Autodesk Inventor part; units mm, degrees
ref_plane "Flange Pattern Plane" through (19.05, 7.9375, -4.5466) normal (0, 1, 0) x (1, 0, 0)
ref_plane "YZ Plane" through (0, 0, 0) normal (1, 0, 0) x (0, 1, 0)
ref_plane "XZ Plane" through (0, 0, 0) normal (0, 1, 0) x (-1, 0, 0)
sketch "Sketch1" plane through (0, 0, 0) normal (0, 1, 0) x (-1, 0, 0)
  line L0 (-19.05, 0) -> (19.05, 0)
  line L1 (19.05, 0) -> (19.05, -25.4)
  line L2 (19.05, -25.4) -> (-19.05, -25.4)
  line L3 (-19.05, -25.4) -> (-19.05, 0)
  line L4 (19.05, 0) -> (-19.05, -25.4) construction
  point P0 (0, 0)
  point P1 (0, 0)
  dimension "d0" = 38.1
  dimension "d1" = 25.4
extrude "Plate1" add sketch "Sketch1" along normal blind 1.5875
sketch "Sketch2" plane through (17.4625, 0, -25.4) normal (1, 0, 0) x (0, 1, 0)
  line L0 (0, 25.4) -> (0, 0)
  line L1 (0, 0) -> (14.2875, 0)
  line L2 (14.2875, 0) -> (14.2875, 25.4)
  line L3 (14.2875, 25.4) -> (0, 25.4)
edge flange "Flanges" height 12.7 angle 90 thickness 1.5875 bend radius 0.7937 thickness toward (1, 0, 0) relief tear relief width 1.5875 relief depth 0.7937 corner gap 1.5875 corner form 0 edges at (19.05, 1.5875, -12.7) (-19.05, 1.5875, -12.7) wall of the first edge with corners at (17.4625, 0, 0) (17.4625, 0, -25.4) (17.4625, 14.2875, -25.4) (17.4625, 14.2875, 0)
bend "Bend1"
corner "Corner1"
sketch "Sketch3" plane through (19.05, 2.3813, -25.4) normal (1, 0, 0) x (0, 0, -1)
  line L0 (-20.8534, 7.8677) -> (-17.2466, 7.8677)
  line L1 (-16.7386, 7.3597) -> (-16.7386, 3.7529)
  line L2 (-17.2466, 3.2449) -> (-20.8534, 3.2449)
  line L3 (-21.3614, 3.7529) -> (-21.3614, 7.3597)
  arc A0 (-20.8534, 7.8677) -> (-21.3614, 7.3597) centre (-20.8534, 7.3597) ccw
  arc A1 (-16.7386, 7.3597) -> (-17.2466, 7.8677) centre (-17.2466, 7.3597) ccw
  arc A2 (-17.2466, 3.2449) -> (-16.7386, 3.7529) centre (-17.2466, 3.7529) ccw
  arc A3 (-21.3614, 3.7529) -> (-20.8534, 3.2449) centre (-20.8534, 3.7529) ccw
  line L4 (-25.4, 0) -> (-25.4, 11.9063) construction
  line L5 (-25.4, 11.9063) -> (0, 11.9062) construction
  line L6 (-20.8534, 7.3597) -> (-17.2466, 3.7529) construction
  point P0 (-25.4, -2.3812)
  point P1 (-16.7386, 3.2449)
  point P2 (-21.3614, 3.2449)
  point P3 (-19.05, 5.5563)
  dimension "d16" = 4.6228
  dimension "d17" = 0.508
  dimension "d20" = 6.35
  dimension "d21" = 6.35
extrude "Flange Stamp" cut sketch "Sketch3" against normal blind 1.5875
sketch "Sketch7" plane through (19.05, 2.3813, 0) normal (1, 0, 0) x (0, 0, -1)
  arc A0 (4.5466, 7.8677) -> (4.0386, 7.3597) centre (4.5466, 7.3597) ccw construction
  arc A1 (8.1534, 3.2449) -> (8.6614, 3.7529) centre (8.1534, 3.7529) ccw construction
  circle A2 centre (6.35, 5.5563) radius 2.1844
  line L0 (4.5466, 7.3597) -> (8.1534, 3.7529) construction
  point P0 (0, -2.3812)
  dimension "d46" = 4.3688
surface extrude "Flange Circle" sketch "Sketch7" against normal up to surface (1.5875 mm away) shown yes curves A2
ref_plane "Flange Pattern Plane" through (19.05, 7.9375, -4.5466) normal (0, 1, 0) x (1, 0, 0)
sketch "Flange Pattern Sketch" plane through (19.05, 7.9375, -4.5466) normal (0, 1, 0) x (1, 0, 0)
  line L0 (0, 3.6068) -> (0, 0) construction
  line L1 (-45.8186, -4.5466) -> (8.2118, -4.5466) construction
  line L2 (0, 0) -> (-1.5875, 0) construction
  point P0 (-19.05, -4.5466)
  point P1 (0, 1.8034)
  point P2 (0, 14.5034)
  dimension "d131" = 12.7
  dimension "d134" = 12.7
pattern_sketch "Flange Pattern" of "Flange Circle", "Flange Stamp" from (19.05, 7.9375, -6.35) copies at (19.05, 7.9375, -19.05)
sketch "Sketch8" plane through (0, 0, 0) normal (0, -1, 0) x (1, 0, 0)
  line L0 (16.6687, 0) -> (-16.6687, 0) construction
  line L1 (14.5034, -4.0386) -> (10.8966, -4.0386)
  line L2 (10.3886, -4.5466) -> (10.3886, -8.1534)
  line L3 (10.8966, -8.6614) -> (14.5034, -8.6614)
  line L4 (15.0114, -8.1534) -> (15.0114, -4.5466)
  arc A0 (15.0114, -4.5466) -> (14.5034, -4.0386) centre (14.5034, -4.5466) ccw
  arc A1 (14.5034, -8.6614) -> (15.0114, -8.1534) centre (14.5034, -8.1534) ccw
  arc A2 (10.3886, -8.1534) -> (10.8966, -8.6614) centre (10.8966, -8.1534) ccw
  arc A3 (10.8966, -4.0386) -> (10.3886, -4.5466) centre (10.8966, -4.5466) ccw
  line L5 (14.5034, -4.5466) -> (10.8966, -8.1534) construction
  line L6 (19.05, 0) -> (19.05, -25.4) construction
  point P0 (0, 0)
  point P1 (10.3886, -8.6614)
  point P2 (15.0114, -8.6614)
  point P3 (12.7, -6.35)
  dimension "d49" = 4.6228
  dimension "d50" = 0.508
  dimension "d51" = 6.35
  dimension "d52" = 6.35
extrude "Body Stamp" cut sketch "Sketch8" against normal blind 1.5875
sketch "Sketch9" plane through (0, 0, 0) normal (0, -1, 0) x (1, 0, 0)
  arc A0 (15.0114, -4.5466) -> (14.5034, -4.0386) centre (14.5034, -4.5466) ccw construction
  arc A1 (10.3886, -8.1534) -> (10.8966, -8.6614) centre (10.8966, -8.1534) ccw construction
  line L0 (14.5034, -4.5466) -> (10.8966, -8.1534) construction
  circle A2 centre (12.7, -6.35) radius 2.1844
  point P0 (0, 0)
  dimension "d55" = 4.3688
surface extrude "Body Circle" sketch "Sketch9" against normal up to surface (1.5875 mm away) shown yes curves A2
sketch "Body Pattern Sketch" plane through (0, 0, 0) normal (0, -1, 0) x (1, 0, 0)
  line L0 (16.6687, 0) -> (-16.6687, 0) construction
  line L1 (19.05, 0) -> (19.05, -25.4) construction
  circle A0 centre (12.7, -6.35) radius 2.1844 construction
  point P0 (0, 0)
  point P1 (12.7, -19.05)
  dimension "d62" = 12.7
  dimension "d65" = 12.7
  dimension "d139" = 12.7
pattern_sketch "Body Pattern" of "Body Stamp", "Body Circle" from (12.7, 0, -6.35) copies at (12.7, 0, -19.05)
sketch "Arc Length" plane through (17.4625, 2.3813, 0) normal (0, 0, 1) x (1, 0, 0)
  line L0 (0, 0) -> (1.5875, 0) construction
  arc A0 (-0.7937, -0.7938) -> (0, 0) centre (-0.7937, 0) ccw construction
  line L1 (-0.7938, -2.3813) -> (-0.7937, -0.7938) construction
  arc A1 (-0.7938, -2.3813) -> (1.5875, 0) centre (-0.7937, 0) ccw construction
  point P0 (-17.4625, -2.3812)
  dimension "d85" = 3.7405
  dimension "d92" = 1.2468
sketch "Sketch13" plane through (19.05, 14.2875, 0) normal (1, 0, 0) x (0, 0, -1)
  line L0 (0, 0) -> (25.4, 0) construction
  line L1 (62.4078, 0) -> (63.4238, -1.016)
  line L2 (63.4238, -1.016) -> (64.4398, 0)
  line L3 (62.4078, 0) -> (64.4398, 0)
  line L4 (25.4, -11.9062) -> (0, -11.9062) construction
  line L5 (63.4238, -10.8903) -> (61.161, -13.1531)
  line L6 (61.161, -13.1531) -> (63.4238, -15.4159)
  line L7 (63.4238, -15.4159) -> (65.6866, -13.1531)
  line L8 (65.6866, -13.1531) -> (63.4238, -10.8903)
  line L9 (63.4238, -10.8903) -> (63.4238, -15.4159) construction
  line L10 (63.4238, -1.016) -> (63.4238, -10.8903) construction
  line L11 (0, -11.9062) -> (25.4, -11.9062) construction
  point P0 (0, -14.2875)
  dimension "d86" = 4.5256
  dimension "d88" = 1.016
  dimension "d91" = 1.016
  dimension "d102" = 63.4238
feature "Notch" [suppressed]
mirror "Notch Mirror" [suppressed]
pattern_linear "Notch Pattern" [suppressed]
chamfer "End Chamfer" distance 1.016 angle 45 4 edges at (-18.2562, 14.2875, -25.4) (18.2563, 14.2875, -25.4) (-18.2562, 14.2875, 0) (18.2562, 14.2875, 0)
sketch "Sketch14" plane through (-19.05, 2.3813, 419.1) normal (1, 0, 0) x (0, 0, -1)
  line L0 (419.1, 11.9063) -> (444.5, 11.9063) construction
  line L1 (419.1, 0) -> (419.1, 11.9063) construction
  line L2 (419.1, -2.3813) -> (444.5, -2.3813) construction
  line L3 (419.1, 11.9063) -> (444.5, 11.9063)
  line L4 (444.5, 11.9063) -> (444.5, -2.3813)
  line L5 (444.5, -2.3813) -> (419.1, -2.3813)
  line L6 (419.1, -2.3813) -> (419.1, 11.9063)
  point P0 (419.1, -2.3812)
  point P1 (382.0521, -1.9844)
extrude "Half Cut" cut sketch "Sketch14" along normal blind 25.4
equation "\"d1\" = 1.27 * Length"
equation "\"d18\" = Thickness"
equation "\"d53\" = Thickness"
equation "\"d89\" = Thickness"
equation "\"d2\" = Thickness"
equation "\"d3\" = BendReliefWidth"
equation "\"d4\" = BendReliefDepth"
equation "\"d5\" = MinimumRemnant"
equation "\"d6\" = TransitionRadius"
equation "\"d10\" = CornerReliefSize"
equation "\"d11\" = GapSize"
equation "\"d12\" = JacobiRadiusSize"
equation "\"BendRadius\" = Thickness"
equation "\"BendReliefWidth\" = Thickness"
equation "\"BendReliefDepth\" = 0.5 * Thickness"
equation "\"CornerReliefSize\" = 4 * Thickness"
equation "\"MinimumRemnant\" = 2 * Thickness"
equation "\"TransitionRadius\" = BendRadius"
equation "\"JacobiRadiusSize\" = BendRadius"
equation "\"GapSize\" = Thickness"
properties part number "Alu C 1x3x1x35"
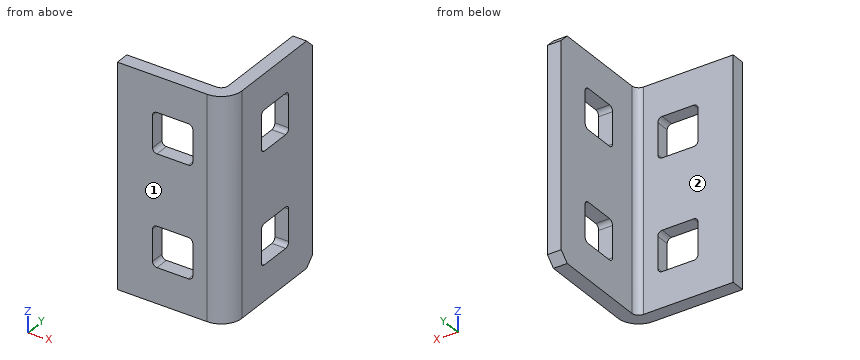
Geometry check sheet. Reference: the model listing, model coordinates, mm. Face numbers are marked on the shaded views. A direction names the side the tool comes from. Round coordinates to 2 decimals unless told otherwise and drop trailing zeros. Loops run counter-clockwise (first coordinate to the right, second up) from the corner with the lowest first, then second, coordinate; pieces in that order, holes last. Notation, with made-up numbers: (-5.5, 10.5) - (41.5, 10.5) arc R7 cw to (41.5, 19.5) - close; hole circle Ø1 at (-36, 16.5). An arc over 180 degrees is marked (long way). Write item = value, one per line. Start each with the question number.
1. Section check D-D on z = -14. Enter the section's corners in (x, y), then the cut area to 3 significant figures.
2. Set-up check for the marked faces 1 and 2: record each of +Z, -Z, +X, -X, +Y, -Y from which the full face is reachable in a straight line by a thin tool's end or side.
3. Section check B-B on z = -7.75. Enter the section's corners in (x, y).
4. Depth check by flat-ended pin: pin 1 (0.5 mm diameter, centred on x = 18, z = -6.5, fed in from -Y); pin 2 (8 mm diameter, centred on y = 9, z = -6.5, fed in from -X); pin 3 (0.5 mm diameter, centred on x = 18, y = 9, fed in from +Z); pin 4 (1.3 mm diameter, centred on y = 1, z = -6.5, fed in from +X). Enter the tip coordinate at first touch or a pass-through.
5. Thickness scan on line 1 (Z direction, x = 17.5, y = 7.5); line 2 (Y direction, x = 12.5, z = -1); line 3 (X direction, y = 4.5, z = -17.5). Record the ranges inside material, lowest first.
6. Section check C-C on y = 8.75. Enter the section's corners in (x, z).
7. Section check A-A on x = 11.5. Enter the section's corners in (y, z), then the cut area to 3 significant figures.
Working result:
q1.outline = (6.35, 0) - (16.67, 0) arc R2.38 ccw to (19.05, 2.38) - (19.05, 14.29) - (17.46, 14.29) - (17.46, 2.38) arc R0.79 cw to (16.67, 1.59) - (6.35, 1.59) - close
q1.area = 39.2 mm^2
q2.face_1 = +Z, -Z, +X, -X, -Y
q2.face_2 = +Z, -Z, -X, +Y
q3.outline = (6.35, 0) - (10.39, 0) - (10.39, 1.59) - (6.35, 1.59) - close; (15.01, 0) - (16.67, 0) arc R2.38 ccw to (19.05, 2.38) - (19.05, 5.63) - (17.46, 5.63) - (17.46, 2.38) arc R0.79 cw to (16.67, 1.59) - (15.01, 1.59) - close; (17.46, 10.25) - (19.05, 10.25) - (19.05, 14.29) - (17.46, 14.29) - close
q4.pin_1 = 0.26
q4.pin_2 = 17.46
q4.pin_3 = 0
q4.pin_4 = 18.93
q5.line_1 = -25.4 to -21.36, -16.74 to -8.66, -4.04 to 0
q5.line_2 = 0 to 1.59
q5.line_3 = 17.46 to 19.05
q6.outline = (17.46, -25.4) - (19.05, -25.4) - (19.05, -21.36) - (17.46, -21.36) - close; (17.46, -16.74) - (19.05, -16.74) - (19.05, -8.66) - (17.46, -8.66) - close; (17.46, -4.04) - (19.05, -4.04) - (19.05, 0) - (17.46, 0) - close
q7.outline = (0, -25.4) - (1.59, -25.4) - (1.59, -21.36) - (0, -21.36) - close; (0, -16.74) - (1.59, -16.74) - (1.59, -8.66) - (0, -8.66) - close; (0, -4.04) - (1.59, -4.04) - (1.59, 0) - (0, 0) - close
q7.area = 25.6 mm^2
